Check sheet for the modelled part. Datum: model origin and axes. Units: mm. A direction names the side the tool comes from. Give positions to 0.01 mm unless a question says otherwise; leave off trailing zeros. Loops run counter-clockwise (first coordinate to the right, second up) from the corner with the lowest first, then second, coordinate; pieces in that order, holes last. Notation, with made-up numbers: (-22.75, -34.75) - (33.25, -34.75) arc R26 cw to (33.25, -8.75) - close; hole circle Ø11 at (59, 44). An arc over 180 degrees is marked (long way). Answer in a Markdown table with one row per item. Add a question column.
(1) Draft check along Y on faces 5 (the face through (0, -12, -1)), 6 (the face through (-0.27, 6.48, -5.53)), 7 (the face through (0, -7.5, -0.5)). Enter one of: released by +Y, released by -Y, zero draft, split by the parting line, or undercut.
(2) Go/stop test with flat-tipped pins: P1, Ø1, axis at y = 5, z = -8, coming from the +X side; P2, Ø6, axis at x = 7.5, y = -9.5, coming from the -Z side; P3, Ø0.9, axis at y = 6.5, z = -15, coming from the -X side. Record where each tip stops, or that it passes through.
(3) Sectioned sample at A-A on z = -6. Enter the section's corners in (x, y), then the cut area to 3 significant figures.
(4) Sectioned sample at C-C on x = 10. Enter the section's corners in (y, z).
(5) Set-up check for faces 1 (the face through (-6.5, 6, -20)), 2 (the face through (-15.5, -5, -1)), 3 (the face through (-12.5, 6, -20)), 4 (the face through (12.5, 6, -20)): record each of +Z, -Z, +X, -X, +Y, -Y from which the full face is reachable in a straight line by a thin tool's end or side.
(6) Sectioned sample at B-B on y = -5. Enter the section's corners in (x, z), then the cut area to 3 significant figures.
(7) Thickness scan on L1, parallel to Z at x = 0, y = 6.6; L2, parallel to X at y = 6.55, z = -33.25; L3, parallel to Z at x = -16, y = -0.5. Record the ranges inside material, lowest first.
(8) Sectioned sample at D-D on x = 0. Enter the section's corners in (y, z).
from build123d import *

# Parameters (mm, degrees)
ESBO_O1_W                         = 40
ESBO_O1_H                         = 20
RESSALTO_EXTRUS_O1_DEPTH          = 1
ESBO_O3_W                         = 40
ESBO_O3_H                         = 20
RESSALTO_EXTRUS_O2_DEPTH          = 2
CORTE_EXTRUS_O1_REACH             = 25.409
CORTE_EXTRUS_O1_DIRECTION_2_REACH = 25.409
ESBO_O4_W                         = 25
ESBO_O4_H                         = 35
ESBO_O4_R                         = 1.25
ESBO_O4_W_2                       = 13
ESBO_O4_H_2                       = 23.5
ESBO_O4_H_3                       = 3
RESSALTO_EXTRUS_O3_DEPTH          = 3
BODY_MOVE_COPY1_START             = 1
BODY_MOVE_COPY1_OUTLINE_W         = 40
BODY_MOVE_COPY1_OUTLINE_H         = 20
BODY_MOVE_COPY1_DEPTH             = 36
BODY_MOVE_COPY1_START_2           = -37
BODY_MOVE_COPY1_2_OUTLINE_W       = 6
BODY_MOVE_COPY1_2_OUTLINE_H       = 3
BODY_MOVE_COPY1_2_DEPTH           = 36
BODY_MOVE_COPY1_START_3           = -2
BODY_MOVE_COPY1_3_DEPTH           = 1
BODY_MOVE_COPY1_START_4           = -8.25
BODY_MOVE_COPY1_4_OUTLINE_W       = 13
BODY_MOVE_COPY1_4_OUTLINE_H       = 3
BODY_MOVE_COPY1_4_DEPTH           = 6.25
BODY_MOVE_COPY1_5_OUTLINE_W       = 13
BODY_MOVE_COPY1_5_OUTLINE_H       = 3
BODY_MOVE_COPY1_5_DEPTH           = 5.25
BODY_MOVE_COPY1_START_5           = 5
BODY_MOVE_COPY1_6_OUTLINE_R       = 1.25
BODY_MOVE_COPY1_6_DEPTH           = 3


with BuildPart() as part:
    # Esboço1 → Ressalto-extrusão1 (new body)
    with BuildSketch(Plane.XY):
        with Locations((0, -2)):
            Rectangle(ESBO_O1_W, ESBO_O1_H)
    extrude(amount=-RESSALTO_EXTRUS_O1_DEPTH)

    # Esboço3 → Ressalto-extrusão2 (add)
    with BuildSketch(Plane.XY):
        with Locations((0, -2)):
            Rectangle(ESBO_O3_W, ESBO_O3_H)
    extrude(amount=RESSALTO_EXTRUS_O2_DEPTH)

    # Corte-extrusão1: up to this face of the body (flat: up to its plane)
    corte_extrus_o1_end = Plane(part.part.faces().sort_by_distance((0, -2, 2))[0])
    # Esboço2 → Corte-extrusão1 (cut, up to the picked face)
    with BuildSketch(Plane.XY, mode=Mode.PRIVATE) as corte_extrus_o1_sk1:
        with BuildLine():
            Line((-2.414021541, -4.35), (-15.5, -4.35))
            Line((-15.5, -4.35), (-15.5, -5.65))
            Line((-15.5, -5.65), (-2.414021541, -5.65))
            ThreePointArc((-2.414021541, -5.65), (0, -7.5), (2.414021541, -5.65))
            Line((2.414021541, -5.65), (15.5, -5.65))
            Line((15.5, -5.65), (15.5, -4.35))
            Line((15.5, -4.35), (2.414021541, -4.35))
            ThreePointArc((2.414021541, -4.35), (0, -2.5), (-2.414021541, -4.35))
        make_face()
    corte_extrus_o1_tool1 = split(extrude(corte_extrus_o1_sk1.sketch, amount=CORTE_EXTRUS_O1_REACH, mode=Mode.PRIVATE), bisect_by=corte_extrus_o1_end, keep=Keep.BOTH, mode=Mode.PRIVATE)
    add(corte_extrus_o1_tool1.solids().sort_by(Axis((0, -5, 0), (0, 0, 1)))[0], mode=Mode.SUBTRACT)

    # Corte-extrusão1 direction 2: up to this face of the body (flat: up to its plane)
    corte_extrus_o1_direction_2_end = Plane(part.part.faces().sort_by_distance((0, -2, -1))[0])
    # Esboço2 → Corte-extrusão1 direction 2 (cut, up to the picked face)
    with BuildSketch(Plane.XY, mode=Mode.PRIVATE) as corte_extrus_o1_direction_2_sk1:
        with BuildLine():
            Line((-2.414021541, -4.35), (-15.5, -4.35))
            Line((-15.5, -4.35), (-15.5, -5.65))
            Line((-15.5, -5.65), (-2.414021541, -5.65))
            ThreePointArc((-2.414021541, -5.65), (0, -7.5), (2.414021541, -5.65))
            Line((2.414021541, -5.65), (15.5, -5.65))
            Line((15.5, -5.65), (15.5, -4.35))
            Line((15.5, -4.35), (2.414021541, -4.35))
            ThreePointArc((2.414021541, -4.35), (0, -2.5), (-2.414021541, -4.35))
        make_face()
    corte_extrus_o1_direction_2_tool1 = split(extrude(corte_extrus_o1_direction_2_sk1.sketch, amount=-CORTE_EXTRUS_O1_DIRECTION_2_REACH, mode=Mode.PRIVATE), bisect_by=corte_extrus_o1_direction_2_end, keep=Keep.BOTH, mode=Mode.PRIVATE)
    add(corte_extrus_o1_direction_2_tool1.solids().sort_by(Axis((0, -5, 0), (0, 0, -1)))[0], mode=Mode.SUBTRACT)

    # Esboço4 → Ressalto-extrusão3 (add)
    # profile 1 of 2: a face of its own
    with BuildSketch(Plane(origin=(0, 8, 0), x_dir=(1, 0, 0), z_dir=(0, 1, 0))):
        with Locations((0, -19.5)):
            Rectangle(ESBO_O4_W, ESBO_O4_H)
        with Locations(Location((0, -33.25, 0), (0, 0, 180))):
            Circle(ESBO_O4_R, mode=Mode.SUBTRACT)
        with Locations((0, -20)):
            Rectangle(ESBO_O4_W_2, ESBO_O4_H_2, mode=Mode.SUBTRACT)
        with Locations(Location((0, -6.75, 0), (0, 0, 180))):
            Circle(ESBO_O4_R, mode=Mode.SUBTRACT)
    # profile 2 of 2: a face of its own
    with BuildSketch(Plane(origin=(0, 8, 0), x_dir=(1, 0, 0), z_dir=(0, 1, 0))):
        with Locations((0, -0.5)):
            Rectangle(ESBO_O4_W, ESBO_O4_H_3)
    extrude(amount=-RESSALTO_EXTRUS_O3_DEPTH)

    # Body-Move/Copy1: read off the stored shape, not the designer's step
    # Body-Move/Copy1 outline → Body-Move/Copy1 (cut)
    with BuildSketch(Plane.XY.offset(BODY_MOVE_COPY1_START)):
        with Locations((0, -2)):
            Rectangle(BODY_MOVE_COPY1_OUTLINE_W, BODY_MOVE_COPY1_OUTLINE_H)
        with BuildLine():
            ThreePointArc((-2.414021541, -4.35), (0, -2.5), (2.414021541, -4.35))
            Line((2.414021541, -4.35), (15.5, -4.35))
            Line((15.5, -4.35), (15.5, -5.65))
            Line((15.5, -5.65), (2.414021541, -5.65))
            ThreePointArc((2.414021541, -5.65), (0, -7.5), (-2.414021541, -5.65))
            Line((-2.414021541, -5.65), (-15.5, -5.65))
            Line((-15.5, -5.65), (-15.5, -4.35))
            Line((-15.5, -4.35), (-2.414021541, -4.35))
        make_face(mode=Mode.SUBTRACT)
    extrude(amount=BODY_MOVE_COPY1_DEPTH, mode=Mode.SUBTRACT)

    # Body-Move_Copy1 2 outline → Body-Move_Copy1 2 (add)
    with BuildSketch(Plane.XY.offset(BODY_MOVE_COPY1_START_2)):
        with Locations((-9.5, 6.5)):
            Rectangle(BODY_MOVE_COPY1_2_OUTLINE_W, BODY_MOVE_COPY1_2_OUTLINE_H)
        with Locations((9.5, 6.5)):
            Rectangle(BODY_MOVE_COPY1_2_OUTLINE_W, BODY_MOVE_COPY1_2_OUTLINE_H)
    extrude(amount=BODY_MOVE_COPY1_2_DEPTH)

    # Body-Move_Copy1 3 outline → Body-Move_Copy1 3 (add)
    with BuildSketch(Plane.XY.offset(BODY_MOVE_COPY1_START_3)):
        Polygon((-20, 8), (-20, -12), (20, -12), (20, 8), (12.5, 8), (12.5, 5), (6.5, 5), (6.5, 8), (-6.5, 8), (-6.5, 5), (-12.5, 5), (-12.5, 8), align=None)
        with BuildLine():
            ThreePointArc((-2.414021541, -4.35), (0, -2.5), (2.414021541, -4.35))
            Line((2.414021541, -4.35), (15.5, -4.35))
            Line((15.5, -4.35), (15.5, -5.65))
            Line((15.5, -5.65), (2.414021541, -5.65))
            ThreePointArc((2.414021541, -5.65), (0, -7.5), (-2.414021541, -5.65))
            Line((-2.414021541, -5.65), (-15.5, -5.65))
            Line((-15.5, -5.65), (-15.5, -4.35))
            Line((-15.5, -4.35), (-2.414021541, -4.35))
        make_face(mode=Mode.SUBTRACT)
    extrude(amount=BODY_MOVE_COPY1_3_DEPTH)

    # Body-Move_Copy1 4 outline → Body-Move_Copy1 4 (add)
    with BuildSketch(Plane.XY.offset(BODY_MOVE_COPY1_START_4)):
        with Locations((0, 6.5)):
            Rectangle(BODY_MOVE_COPY1_4_OUTLINE_W, BODY_MOVE_COPY1_4_OUTLINE_H)
    extrude(amount=BODY_MOVE_COPY1_4_DEPTH)

    # Body-Move_Copy1 5 outline → Body-Move_Copy1 5 (add)
    with BuildSketch(Plane.XY.offset(BODY_MOVE_COPY1_START_2)):
        with Locations((0, 6.5)):
            Rectangle(BODY_MOVE_COPY1_5_OUTLINE_W, BODY_MOVE_COPY1_5_OUTLINE_H)
    extrude(amount=BODY_MOVE_COPY1_5_DEPTH)

    # Body-Move_Copy1 6 outline → Body-Move_Copy1 6 (cut)
    with BuildSketch(Plane(origin=(0, 0, 0), x_dir=(1, 0, 0), z_dir=(0, 1, 0)).offset(BODY_MOVE_COPY1_START_5)):
        with Locations((0, 6.75)):
            Circle(BODY_MOVE_COPY1_6_OUTLINE_R)
        with Locations((0, 33.25)):
            Circle(BODY_MOVE_COPY1_6_OUTLINE_R)
    extrude(amount=BODY_MOVE_COPY1_6_DEPTH, mode=Mode.SUBTRACT)


solid = part.part
Reply:
| question | item | result |
|---|---|---|
| 1 | face 5 | released by -Y |
| 1 | face 6 | zero draft |
| 1 | face 7 | undercut |
| 2 | P1 | x = 12.5 |
| 2 | P2 | z = -2 |
| 2 | P3 | x = -12.5 |
| 3 | outline | (-12.5, 5) - (-1, 5) - (-1, 8) - (-12.5, 8) - close; (1, 5) - (12.5, 5) - (12.5, 8) - (1, 8) - close |
| 3 | area | 69.0 mm^2 |
| 4 | outline | (-12, -2) - (-5.65, -2) - (-5.65, 1) - (-12, 1) - close; (-4.35, -2) - (5, -2) - (5, -37) - (8, -37) - (8, 1) - (-4.35, 1) - close |
| 5 | face 1 | +Y, -Y |
| 5 | face 2 | +Z, -Z |
| 5 | face 3 | -Z, -X, +Y, -Y |
| 5 | face 4 | -Z, +X, +Y, -Y |
| 6 | outline | (-20, -2) - (-15.5, -2) - (-15.5, 1) - (-20, 1) - close; (15.5, -2) - (20, -2) - (20, 1) - (15.5, 1) - close |
| 6 | area | 27.0 mm^2 |
| 7 | L1 | -37 to -34.5, -32 to -31.75, -8.25 to -8, -5.5 to 1 |
| 7 | L2 | -12.5 to -1.25, 1.25 to 12.5 |
| 7 | L3 | -2 to 1 |
| 8 | outline | (-12, -2) - (-7.5, -2) - (-7.5, 1) - (-12, 1) - close; (-2.5, -2) - (5, -2) - (5, -5.5) - (8, -5.5) - (8, 1) - (-2.5, 1) - close; (5, -37) - (8, -37) - (8, -34.5) - (5, -34.5) - close; (5, -32) - (8, -32) - (8, -31.75) - (5, -31.75) - close; (5, -8.25) - (8, -8.25) - (8, -8) - (5, -8) - close |
